Build history of the part. All positions in model axes, mm. Give positions to 0.01 mm unless a question says otherwise; leave off trailing zeros. Write each loop counter-clockwise with the first axis right and the second up, starting at its lowest first coordinate (ties: lowest second). Pieces come first, ordered by that corner, then holes. Notation, with made-up numbers: (75.5, -28.75) -> (120.5, -28.75) arc R20 cw to (120.5, -14.75) -> close; hole circle Ø11 at (10, 52.5). An arc over 180 degrees is marked (long way). One line per question, with ' | ' between items. Start each with the question number.
(1) Band-saw the part on C-C, the plane y = 0.5. Count the separate pieces of the cut face and the enclosed holes in it, and give its area (3 significant figures).
(2) Band-saw the part on A-A, the plane z = 0. Give the cut face in (x, y) (3 decimals), and give its area (3 significant figures).
(3) Band-saw the part on B-B, the plane x = -53.34. Give the cut face in (y, z) (3 decimals), and give its area (3 significant figures).
(4) Pin check, flat tips, straight feed: P1, Ø3, axis at x = 8.5, z = -38, coming from the -Y side (3 decimals); P2, Ø3, axis at y = 1, z = -27, coming from the +X side; P3, Ø2, axis at x = -41, y = -2, coming from the -Z side. Stop position of each tip, or through.
(5) Pull direction Z, two halves, no side cores. Call faces 1 (the flat face through (-25.68, 0.04, 33.84)), 2 (the cylindrical face through (59.688, 0.044, -0.206)): released by +Z, released by -Z, zero draft, split by the parting line, or undercut.
(6) Drill centre lines: probe 1 along X at (y, z) = (-2.25, 44.5); probe 2 along Z at (x, y) = (38, 1.25); probe 3 along Z at (x, y) = (-36, -1.25). Where is each one in solid material? Low to high. Write a range as from..to.
from build123d import *

# Parameters (mm, degrees)
BOSS_EXTRUDE1_DEPTH = 3.175
CIRPATTERN4_COUNT   = 19
FILLET1_R           = 2.54
BOSS_EXTRUDE2_DEPTH = 6.35
SKETCH7_R           = 3.175
CUT_EXTRUDE3_DEPTH  = 6.35
CIRPATTERN5_COUNT   = 6


with BuildPart() as part:
    # Sketch1 → Boss-Extrude1 (new, symmetric)
    with BuildSketch(Plane(origin=(0, 0, 0), x_dir=(1, 0, 0), z_dir=(0, 1, 0))):
        with BuildLine():
            Line((40.994673778, 3.120969289), (49.927314923, 9.375671955))
            ThreePointArc((49.927314923, 9.375671955), (50.8, 0), (49.927314923, -9.375671955))
            Line((49.927314923, -9.375671955), (40.994673778, -3.120969289))
            ThreePointArc((40.994673778, -3.120969289), (39.37, 0), (40.994673778, 3.120969289))
        make_face()
    boss_extrude1 = extrude(amount=BOSS_EXTRUDE1_DEPTH, both=True)

    # CirPattern4: Boss-Extrude1 ×19 about axis
    cirpattern4_axis = Axis((0, 0, 0), (0, 1, 0))
    for i in range(1, CIRPATTERN4_COUNT):
        add(boss_extrude1.rotate(cirpattern4_axis, i * 360 / CIRPATTERN4_COUNT))

    # Fillet1
    fillet1_edges = [part.edges().sort_by_distance(p)[0] for p in [
        (47.969309878, 0, 8.004662063),
        (47.969309878, 0, -8.004662063),
        (42.771090832, 0, 23.146556848),
        (32.937960433, 0, 35.780163044),
        (19.535490936, 0, 44.536433387),
        (4.016047871, 0, 48.466490119),
        (-11.938596296, 0, 47.144450611),
        (-26.599508308, 0, 40.713578358),
        (-38.37795086, 0, 29.870758154),
        (-45.997546942, 0, 15.790977811),
        (-48.632595087, 0, 0),
        (-45.997546942, 0, -15.790977811),
        (-38.37795086, 0, -29.870758154),
        (-26.599508308, 0, -40.713578358),
        (-11.938596296, 0, -47.144450611),
        (4.016047871, 0, -48.466490119),
        (19.535490936, 0, -44.536433387),
        (32.937960433, 0, -35.780163044),
        (42.771090832, 0, -23.146556848),
    ]]
    fillet(fillet1_edges, radius=FILLET1_R)

    # Sketch5 → Boss-Extrude2 (add)
    with BuildSketch(Plane(origin=(0, 3.175, 0), x_dir=(1, 0, 0), z_dir=(0, 1, 0))):
        with BuildLine():
            Line((50.022125, -8.855902579), (45.72, 0))
            Line((45.72, 0), (50.022125, 8.855902579))
            ThreePointArc((50.022125, 8.855902579), (59.69, 0), (50.022125, -8.855902579))
        make_face()
    boss_extrude2 = extrude(amount=-BOSS_EXTRUDE2_DEPTH)

    # Sketch7 → Cut-Extrude3 (cut)
    with BuildSketch(Plane(origin=(0, 3.175, 0), x_dir=(1, 0, 0), z_dir=(0, 1, 0))):
        with Locations(Location((53.34, 0, 0), (0, 0, 270))):
            Circle(SKETCH7_R)
    cut_extrude3 = extrude(amount=-CUT_EXTRUDE3_DEPTH, mode=Mode.SUBTRACT)

    # CirPattern5: Boss-Extrude2, Cut-Extrude3 ×6 about axis
    cirpattern5_axis = Axis((0, 0, 0), (0, 1, 0))
    add([boss_extrude2.rotate(cirpattern5_axis, i * 360 / CIRPATTERN5_COUNT) for i in range(1, CIRPATTERN5_COUNT)])
    add([cut_extrude3.rotate(cirpattern5_axis, i * 360 / CIRPATTERN5_COUNT) for i in range(1, CIRPATTERN5_COUNT)], mode=Mode.SUBTRACT)


solid = part.part
Results:
1) separate pieces: 1 | enclosed holes: 7 | area: 3,120 mm²
2) outline: (-59.69, -3.175) -> (-56.515, -3.175) -> (-56.515, 3.175) -> (-59.69, 3.175) -> close; (-50.165, -3.175) -> (-45.278, -3.175) -> (-45.278, 3.175) -> (-50.165, 3.175) -> close; (39.37, -3.175) -> (50.165, -3.175) -> (50.165, 3.175) -> (39.37, 3.175) -> close; (56.515, -3.175) -> (59.69, -3.175) -> (59.69, 3.175) -> (56.515, 3.175) -> close | area: 140 mm²
3) outline: (-3.175, -8.519) -> (3.175, -8.519) -> (3.175, -3.175) -> (-3.175, -3.175) -> close; (-3.175, 3.175) -> (3.175, 3.175) -> (3.175, 8.519) -> (-3.175, 8.519) -> close | area: 67.9 mm²
4) P1: stops at y = -3.175 | P2: stops at x = 43.94 | P3: stops at z = -31.32
5) face 1: undercut | face 2: split by the parting line
6) probe 1: x = -34.28..-29.36, -23.98..1.85, 5.21..23.98, 29.36..34.28 | probe 2: z = -33.71..-22.85, -16.59..-11.48, 11.48..16.59, 22.85..33.71 | probe 3: z = -35.84..-27.38, -25.12..-17.29, 17.29..25.12, 27.38..35.84
